```python
from build123d import *

# Parameters (mm, degrees)
F0_R     = 11
F1_DEPTH = 2
F2_W     = 9
F2_H     = 3
F2_W_2   = 3
F2_H_2   = 9
F3_DEPTH = 1
F4_W     = 1.5
F4_H     = 3
F4_W_2   = 3
F4_H_2   = 1.5
F5_DEPTH = 75
F6_W     = 3
F6_H     = 9
F6_W_2   = 9
F6_H_2   = 3
F7_DEPTH = 2


with BuildPart() as f1:
    # F0 (on Top) → F1 (new body)
    with BuildSketch(Plane.XY):
        Circle(F0_R)
    extrude(amount=F1_DEPTH)

    # F2 (on face) → F3 (join)
    with BuildSketch(Plane.XY.offset(2)):
        with Locations((-6, 0)):
            Rectangle(F2_W, F2_H)
        with Locations((6, 0)):
            Rectangle(F2_W, F2_H)
        with Locations((0, 6)):
            Rectangle(F2_W_2, F2_H_2)
        with Locations((0, -6)):
            Rectangle(F2_W_2, F2_H_2)
    extrude(amount=F3_DEPTH)

    # F4 (on face) → F5 (join)
    with BuildSketch(Plane.XY.offset(2)):
        with Locations((9.75, 0)):
            Rectangle(F4_W, F4_H)
        Polygon((8, -1.5), (8, 1.5), (8, 2.5), (6, 2.5), (6, 1.5), (6, -1.5), (6, -2.5), (8, -2.5), align=None)
        Polygon((5, -1.5), (5, 1.5), (5, 2.5), (3, 2.5), (3, 1.5), (3, -1.5), (3, -2.5), (5, -2.5), align=None)
        Polygon((2, -1.5), (2, 1.5), (1.5, 1.5), (1.5, 2), (-1.5, 2), (-1.5, 1.5), (-2, 1.5), (-2, -1.5), (-1.5, -1.5), (-1.5, -2), (1.5, -2), (1.5, -1.5), align=None)
        Polygon((2.5, 6), (2.5, 8), (1.5, 8), (-1.5, 8), (-2.5, 8), (-2.5, 6), (-1.5, 6), (1.5, 6), align=None)
        Polygon((2.5, 3), (2.5, 5), (1.5, 5), (-1.5, 5), (-2.5, 5), (-2.5, 3), (-1.5, 3), (1.5, 3), align=None)
        with Locations((0, 9.75)):
            Rectangle(F4_W_2, F4_H_2)
        Polygon((-6, 2.5), (-8, 2.5), (-8, 1.5), (-8, -1.5), (-8, -2.5), (-6, -2.5), (-6, -1.5), (-6, 1.5), align=None)
        Polygon((-3, 2.5), (-5, 2.5), (-5, 1.5), (-5, -1.5), (-5, -2.5), (-3, -2.5), (-3, -1.5), (-3, 1.5), align=None)
        with Locations((-9.75, 0)):
            Rectangle(F4_W, F4_H)
        Polygon((-2.5, -6), (-2.5, -8), (-1.5, -8), (1.5, -8), (2.5, -8), (2.5, -6), (1.5, -6), (-1.5, -6), align=None)
        Polygon((-2.5, -3), (-2.5, -5), (-1.5, -5), (1.5, -5), (2.5, -5), (2.5, -3), (1.5, -3), (-1.5, -3), align=None)
        with Locations((0, -9.75)):
            Rectangle(F4_W_2, F4_H_2)
    extrude(amount=F5_DEPTH)

    # F6 (on face) → F7 (join)
    with BuildSketch(Plane.XY.offset(77)):
        with Locations((0, 6)):
            Rectangle(F6_W, F6_H)
        with Locations((-6, 0)):
            Rectangle(F6_W_2, F6_H_2)
        with Locations((0, -6)):
            Rectangle(F6_W, F6_H)
        with Locations((6, 0)):
            Rectangle(F6_W_2, F6_H_2)
    extrude(amount=-F7_DEPTH)


solid = f1.part
```
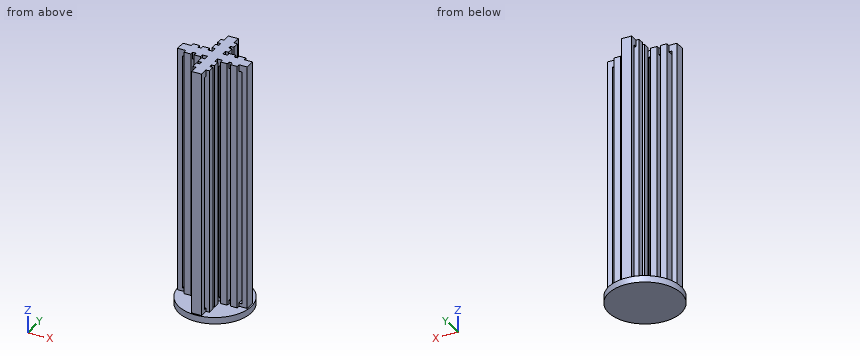
The listing builds one solid part. Answer for the finished solid, in the listing's coordinates (mm). Coordinates: 2 decimals unless noted, no trailing zeros. Write item = value, one per line.
1) Section A-A (y = 0) is taken. Count the separate pieces of the cut face and the enclosed holes in it, plus the area to 3 significant figures.
Responses:
separate_pieces = 1
enclosed_holes = 6
area = 1,190 mm^2
2) Find the intervals of material crossed by line 1 along Z through (x, y) = (0.25, 8.75); line 2 along X through (y, z) = (-7.5, 27); line 3 along Z through (x, y) = (-2, 2.25), in increasing order.
Responses:
line_1 = 0 to 3, 75 to 77
line_2 = -2.5 to 2.5
line_3 = 0 to 2
3) Each of these flat-tipped pins is pushed along its axis until it touches: P1, Ø1, axis at x = -2.5, z = 64, coming from the +Y side; P2, Ø0.6, axis at x = 7, z = 36.5, coming from the -Y side; P3, Ø2.5, axis at x = 1, z = 57.5, coming from the +Y side; P4, Ø6, axis at x = 4.5, y = -3.5, coming from the -Z side. Where does it stop, or does it pass through?
Responses:
P1 = 8
P2 = -2.5
P3 = 10.5
P4 = 0
